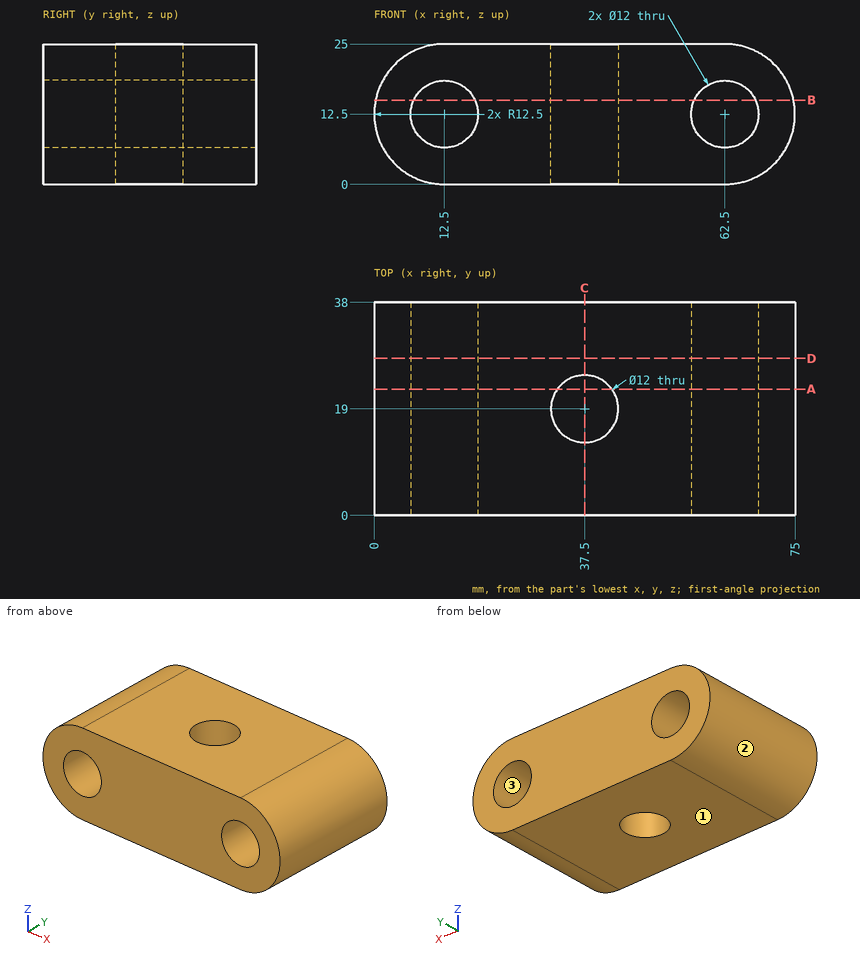
Geometry: see drawing. Coordinates: mm, zero at the bounding-box minimum. Coordinates: 2 decimals unless noted, no trailing zeros. Loops run counter-clockwise (first coordinate to the right, second up) from the corner with the lowest first, then second, coordinate; pieces in that order, holes last. Notation, with made-up numbers: M 79,58.5 L 83,58.5 A21 cw 83,73.5 Z; hole C -2.75,37.5 d10. An arc over 180 degrees is marked long. Answer in a Markdown table with one row per item.
Q1. First-contact query: pin 1 (3 mm diameter, centred on y = 15, z = 15, fed in from -X). Flat tip, straight axial feed; report the tip coordinate or a pass-through.
Answers below:
| item | result |
|---|---|
| pin 1 | stops at x = 0.04 |
Q2. Section C-C on x = 37.5. Return the cut outline in (y, z).
Answers below:
| item | result |
|---|---|
| outline | M 0,0 L 13,0 L 13,25 L 0,25 Z; M 25,0 L 38,0 L 38,25 L 25,25 Z |
Q3. Draft query along X for the marked faces 1, 2 and 3. Return one class per face: pulls with the +X half, pulls with the -X half, needs draft (parallel to the pull), parting line crosses it, or undercut.
Answers below:
| item | result |
|---|---|
| face 1 | needs draft |
| face 2 | pulls with the -X half |
| face 3 | undercut |
Q4. Section D-D on y = 28. Return the cut outline in (x, z).
Answers below:
| item | result |
|---|---|
| outline | M 12.5,0 L 62.5,0 A12.5 ccw 62.5,25 L 12.5,25 A12.5 ccw Z; hole C 12.5,12.5 d12; hole C 62.5,12.5 d12 |
Q5. Section B-B on z = 15. Return the cut outline in (x, y), plus the area to 3 significant figures.
Answers below:
| item | result |
|---|---|
| outline | M 0.25,0 L 7.05,0 L 7.05,38 L 0.25,38 Z; M 17.95,0 L 57.05,0 L 57.05,38 L 17.95,38 Z; M 67.95,0 L 74.75,0 L 74.75,38 L 67.95,38 Z; hole C 37.5,19 d12 |
| area | 1,890 mm^2 |
Q6. Section A-A on y = 22.5. Return the cut outline in (x, z).
Answers below:
| item | result |
|---|---|
| outline | M 12.5,0 L 32.63,0 L 32.63,25 L 12.5,25 A12.5 ccw Z; M 42.37,0 L 62.5,0 A12.5 ccw 62.5,25 L 42.37,25 Z; hole C 12.5,12.5 d12; hole C 62.5,12.5 d12 |
Q7. Ray query, probe 1 along Z at (x, y) = (62.5, 27); probe 2 along X at (y, z) = (29, 12); probe 3 along X at (y, z) = (17, 9.75). Return the intervals inside material, ascending. Write a range as from..to.
Answers below:
| item | result |
|---|---|
| probe 1 | z = 0..6.5, 18.5..25 |
| probe 2 | x = 0.01..6.52, 18.48..56.52, 68.48..74.99 |
| probe 3 | x = 0.31..7.17, 17.83..31.84, 43.16..57.17, 67.83..74.69 |
